Geometry check sheet. Reference: drawing and pictorial views, mm from the part's lowest x, y, z. Coordinates: 2 decimals unless noted, no trailing zeros. Write each loop counter-clockwise with the first axis right and the second up, starting at its lowest first coordinate (ties: lowest second). Pieces come first, ordered by that corner, then holes. Notation, with made-up numbers: (-6, 1) - (13, 1) arc R17 cw to (13, 8) - close; hole circle Ø5 at (8.5, -19.5). An arc over 180 degrees is marked (long way). Answer as a JSON object with one key per item and string values. Group by question number.
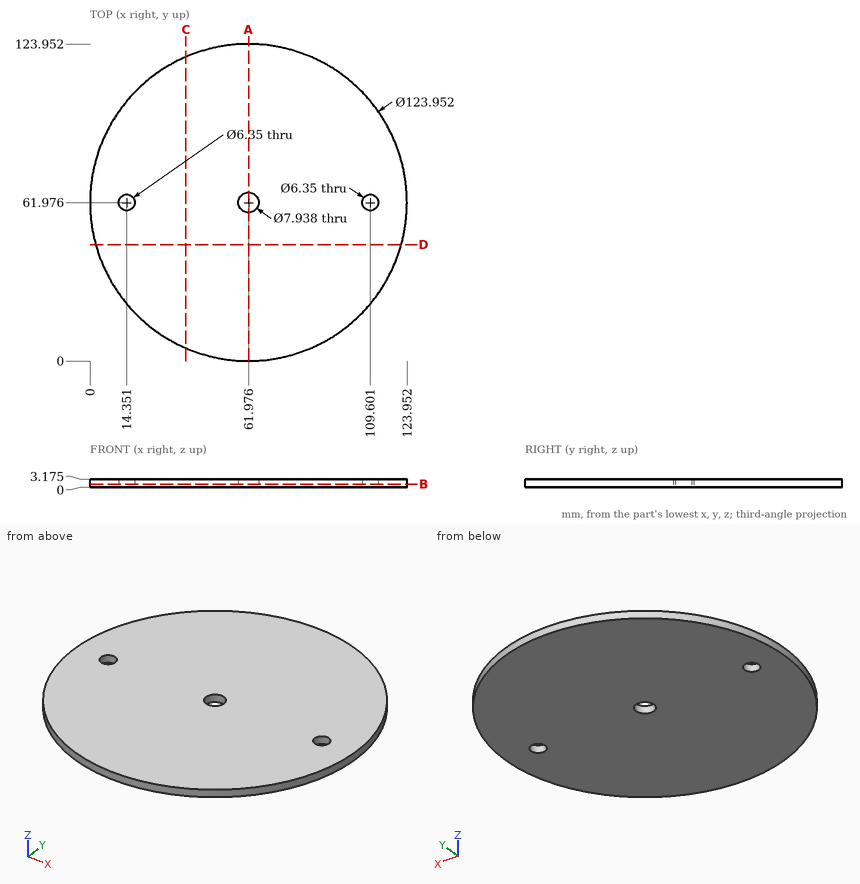
(1) Section check A-A (x = 62). Record the cut outline in (y, z) (1 decimal).
(2) Section check B-B (z = 1.2). Count the separate pieces of the cut face and the enclosed holes in it, and give its area (3 significant figures).
(3) Gauge pin test, flat ends, axial feed: pin 1 (1 mm diameter, centred on y = 14.5, z = 2, fed in from +X); pin 2 (1.5 mm diameter, centred on y = 67, z = 2, fed in from +X) (1 decimal). Record the tip position at first contact, or that the pin passes through.
(4) Section check C-C (x = 37.5). Record the cut outline in (y, z) (1 decimal).
(5) Material ranges on L1, parallel to Y at x = 62, z = 1.85 (1 decimal); L2, parallel to X at y = 61, z = 1.55 (1 decimal); L3, parallel to Y at x = 111.5, z = 1.7 (1 decimal), recorded low to high. Write a range as [from, to].
(6) Section check D-D (y = 45.5). Record the cut outline in (x, z) (1 decimal).
Conclusion:
{
 "1": {"outline": "(0, 0) - (58, 0) - (58, 3.2) - (0, 3.2) - close; (65.9, 0) - (124, 0) - (124, 3.2) - (65.9, 3.2) - close"},
 "2": {"separate pieces": "1", "enclosed holes": "3", "area": "12,000 mm^2"},
 "3": {"pin 1": "stops at x = 102.4", "pin 2": "stops at x = 123.8"},
 "4": {"outline": "(5, 0) - (118.9, 0) - (118.9, 3.2) - (5, 3.2) - close"},
 "5": {"L1": "y = [0, 58], [65.9, 124]", "L2": "x = [0, 11.3], [17.4, 58.1], [65.8, 106.6], [112.6, 123.9]", "L3": "y = [24.7, 59.4], [64.5, 99.2]"},
 "6": {"outline": "(2.2, 0) - (121.7, 0) - (121.7, 3.2) - (2.2, 3.2) - close"}
}
